```python
from build123d import *

# Parameters (mm, degrees)
BOSS_EXTRUDE1_DEPTH = 1.9
SKETCH2_R           = 1.5
CUT_EXTRUDE1_DEPTH  = 2.3
FILLET1_R           = 0.3


with BuildPart() as part:
    # Sketch1 → Boss-Extrude1 (new body)
    with BuildSketch(Plane(origin=(0, 0, 0), x_dir=(1, 0, 0), z_dir=(0, 1, 0))):
        Polygon((1.732050808, -3), (3.464101615, 0), (1.732050808, 3), (-1.732050808, 3), (-3.464101615, 0), (-1.732050808, -3), align=None)
    extrude(amount=BOSS_EXTRUDE1_DEPTH)

    # Sketch2 → Cut-Extrude1 (cut)
    with BuildSketch(Plane(origin=(0, 1.9, 0), x_dir=(1, 0, 0), z_dir=(0, 1, 0))):
        with Locations(Location((0, 0, 0), (0, 0, 270))):
            Circle(SKETCH2_R)
    extrude(amount=-CUT_EXTRUDE1_DEPTH, mode=Mode.SUBTRACT)

    # Fillet1
    fillet1_edges = [part.edges().sort_by_distance(p)[0] for p in [
        (2.598076211, 1.9, -1.5),
        (0, 1.9, -3),
        (-2.598076211, 1.9, -1.5),
        (-2.598076211, 1.9, 1.5),
        (0, 1.9, 3),
        (-2.598076211, 0, 1.5),
        (-2.598076211, 0, -1.5),
        (0, 0, -3),
        (2.598076211, 0, -1.5),
        (2.598076211, 0, 1.5),
        (0, 0, 3),
        (2.598076211, 1.9, 1.5),
    ]]
    fillet(fillet1_edges, radius=FILLET1_R)


solid = part.part
```
For this review, take the finished solid that the model builds, in its own axes (mm). Coordinates: 2 decimals unless noted, no trailing zeros. Order: outer loops, then holes, each group sorted by start corner. A loop starts at its lowest first (then second) coordinate and runs counter-clockwise, first axis right, second up. Notation, with made-up numbers: (-38, -30) -> (-10, -30) arc R37 ccw to (-10, 7) -> close; hole circle Ø1 at (61, 35). An arc over 180 degrees is marked (long way). Use CSV: the item, a comma, the result in double quotes. Start each with the question number.
Item 1: We need section C-C, the plane y = 1.75. Give the boundary of the cut face in (x, z), then the cut area to 3 significant figures.
Item 2: We need section B-B, the plane y = 1.3. Give the boundary of the cut face in (x, z).
Item 3: Wall thickness on probe 1 along Z at (x, y) = (1, 1.35); probe 2 along Z at (x, y) = (0.25, 0.3); probe 3 along X at (y, z) = (1.6, -1.25): over which ranges is each line inside the solid? List them lowest first.
Item 4: We need section D-D, the plane x = -1.25. Give the boundary of the cut face in (y, z).
Item 5: We need section A-A, the plane x = 0. Give the boundary of the cut face in (y, z).
Item 6: Draft analysis for pull direction X (two halves, no side actions). For faces 1 (the face through (2.51, 1.81, -1.48)), 2 (the face through (1.3, 0, -1.2)), 3 (the face through (0.45, 0.96, 1.43)), 4 (the face through (-2.532, 1.814, -1.434)), state which applies: pulls with the +X half, pulls with the -X half, needs draft (parallel to the pull), parting line crosses it, or undercut.
Derived:
1,outline,"(-3.42, 0) -> (-1.71, -2.96) -> (1.71, -2.96) -> (3.42, 0) -> (1.71, 2.96) -> (-1.71, 2.96) -> close; hole circle Ø3 at (0, 0)"
1,area,"23.3 mm^2"
2,outline,"(-3.46, 0) -> (-1.73, -3) -> (1.73, -3) -> (3.46, 0) -> (1.73, 3) -> (-1.73, 3) -> close; hole circle Ø3 at (0, 0)"
3,probe 1,"z = -3 to -1.12, 1.12 to 3"
3,probe 2,"z = -3 to -1.48, 1.48 to 3"
3,probe 3,"x = -2.74 to -0.83, 0.83 to 2.74"
4,outline,"(0, -2.7) arc R0.3 ccw to (0.3, -3) -> (1.6, -3) arc R0.3 ccw to (1.9, -2.7) -> (1.9, -0.83) -> (0, -0.83) -> close; (0, 0.83) -> (1.9, 0.83) -> (1.9, 2.7) arc R0.3 ccw to (1.6, 3) -> (0.3, 3) arc R0.3 ccw to (0, 2.7) -> close"
5,outline,"(0, -2.7) arc R0.3 ccw to (0.3, -3) -> (1.6, -3) arc R0.3 ccw to (1.9, -2.7) -> (1.9, -1.5) -> (0, -1.5) -> close; (0, 1.5) -> (1.9, 1.5) -> (1.9, 2.7) arc R0.3 ccw to (1.6, 3) -> (0.3, 3) arc R0.3 ccw to (0, 2.7) -> close"
6,face 1,"pulls with the +X half"
6,face 2,"needs draft"
6,face 3,"undercut"
6,face 4,"pulls with the -X half"
